```python
from build123d import *

# Parameters (mm, degrees)
SKETCH1_R           = 3
SKETCH1_R_2         = 1.5
BOSS_EXTRUDE1_DEPTH = 100
SKETCH2_R           = 1.5
BOSS_EXTRUDE2_DEPTH = 10


with BuildPart() as part:
    # Sketch1 → Boss-Extrude1 (new body)
    with BuildSketch(Plane.XY):
        Circle(SKETCH1_R)
        Circle(SKETCH1_R_2, mode=Mode.SUBTRACT)
    extrude(amount=BOSS_EXTRUDE1_DEPTH)

    # Sketch2 → Boss-Extrude2 (add)
    with BuildSketch(Plane.XY.offset(100)):
        Polygon((4.618802154, 0), (2.309401077, 4), (-2.309401077, 4), (-4.618802154, 0), (-2.309401077, -4), (2.309401077, -4), align=None)
        Circle(SKETCH2_R, mode=Mode.SUBTRACT)
    boss_extrude2 = extrude(amount=-BOSS_EXTRUDE2_DEPTH)

    # Mirror1: Boss-Extrude2 across plane
    add(boss_extrude2.mirror(Plane.XY.offset(50)))


solid = part.part
```
The listing builds one solid part. Answer for the finished solid, in the listing's coordinates (mm). A direction names the side the tool comes from. Coordinates: 2 decimals unless noted, no trailing zeros. Write each loop counter-clockwise with the first axis right and the second up, starting at its lowest first coordinate (ties: lowest second). Pieces come first, ordered by that corner, then holes. Notation, with made-up numbers: M -35,-8.75 L 10,-8.75 A16 ccw 10,16.25 Z; hole C -29,-5 d3. An arc over 180 degrees is marked long. Use a Markdown table: item, result. Add a question column.
1. For a pull along Z with two mould halves and no side action, classify faces 3 (the cylindrical face through (-1.5, 0.07, 49.3)), 4 (the cylindrical face through (-3, 0, 49)), 5 (the flat face through (2, 0, 0)) as +Z half, -Z half, draft (parallel to the pull), parting line (faces both ways), or undercut.
2. Section C-C (z = 53.5) is taken. Give the vertices of the cut face in (x, y), plus the area to 3 significant figures.
3. Section A-A (x = 0.5) is taken. Give the vertices of the cut face in (y, z).
4. Straight lines are drawn through the part: line 1 along Y through (x, z) = (0, 26.5); line 2 along Z through (x, y) = (3.75, 1.25); line 3 along Y through (x, z) = (1, 61). For each, find the intervals that lie inside material, in ascending order. Write a range as [from, to].
5. Which of the six approach directions +Z, -Z, +X, -X, +Y, -Y give full straight-line access (tool end or side, diameter ignored) to faces 1 (the flat face through (3, 1, 90)), 2 (the flat face through (-3.48, -1.97, 4.93))?
6. Section B-B (z = 94.5) is taken. Give the vertices of the cut face in (x, y), plus the area to 3 significant figures.
7. Given P1, Ø1.5, axis at y = -2, z = 24, coming from the +X side; P2, Ø4, axis at y = -1.5, z = 23, coming from the -X side; P3, Ø1.5, axis at x = 2.5, y = -2.5, coming from the -Z side; P4, Ø1, axis at y = 1, z = 61.5, coming from the +X side, each flat-ended and moving along its own axis, determine where each tip first touches the part or whether it passes through.
Data:
| question | item | result |
|---|---|---|
| 1 | face 3 | draft |
| 1 | face 4 | undercut |
| 1 | face 5 | -Z half |
| 2 | outline | C 0,0 d6; hole C 0,0 d3 |
| 2 | area | 21.2 mm2 |
| 3 | outline | M -4,0 L -1.41,0 L -1.41,100 L -4,100 L -4,90 L -2.96,90 L -2.96,10 L -4,10 Z; M 1.41,0 L 4,0 L 4,10 L 2.96,10 L 2.96,90 L 4,90 L 4,100 L 1.41,100 Z |
| 4 | line 1 | y = [-3, -1.5], [1.5, 3] |
| 4 | line 2 | z = [0, 10], [90, 100] |
| 4 | line 3 | y = [-2.83, -1.12], [1.12, 2.83] |
| 5 | face 1 | none |
| 5 | face 2 | +Z, -Z, -X, -Y |
| 6 | outline | M -4.62,0 L -2.31,-4 L 2.31,-4 L 4.62,0 L 2.31,4 L -2.31,4 Z; hole C 0,0 d3 |
| 6 | area | 48.4 mm2 |
| 7 | P1 | stops at x = 2.73 |
| 7 | P2 | stops at x = -3 |
| 7 | P3 | stops at z = 0 |
| 7 | P4 | stops at x = 2.96 |
